from build123d import *

# Parameters (mm, degrees)
SKETCH1_W          = 110
SKETCH1_H          = 25
SKETCH2_W          = 16
SKETCH2_H          = 11.86901723
CUT_EXTRUDE1_DEPTH = 90
CHAMFER1_SIZE      = 2
FILLET1_R          = 3


with BuildPart() as part:
    # Sketch1 → Revolve1 (revolve)
    with BuildSketch(Plane.XY, mode=Mode.PRIVATE) as revolve1_sk:
        with Locations((0, 12.5)):
            Rectangle(SKETCH1_W, SKETCH1_H)
    revolve(revolve1_sk.sketch.rotate(Axis((-55, 0, 0), (1, 0, 0)), 90), axis=Axis((-55, 0, 0), (1, 0, 0)))

    # Sketch2 → Cut-Extrude1 (cut)
    with BuildSketch(Plane(origin=(55, 0, 0), x_dir=(0, 0, -1), z_dir=(1, 0, 0))):
        with Locations((0, 24.934508615)):
            Rectangle(SKETCH2_W, SKETCH2_H)
    extrude(amount=-CUT_EXTRUDE1_DEPTH, mode=Mode.SUBTRACT)

    # Chamfer1
    chamfer1_edges = [part.edges().sort_by_distance(p)[0] for p in [
        (55, -20.310096012, -14.577379737),
    ]]
    chamfer(chamfer1_edges, length=CHAMFER1_SIZE)

    # Fillet1
    fillet1_edges = [part.edges().sort_by_distance(p)[0] for p in [
        (-35, 19, 0),
    ]]
    fillet(fillet1_edges, radius=FILLET1_R)


solid = part.part
Build history of the part. All positions in model axes, mm. A direction names the side the tool comes from. Coordinates: 2 decimals unless noted, no trailing zeros. Write each loop counter-clockwise with the first axis right and the second up, starting at its lowest first coordinate (ties: lowest second). Pieces come first, ordered by that corner, then holes. Notation, with made-up numbers: (32, 0.25) -> (38, 0.25) arc R23 cw to (38, 8.25) -> close; hole circle Ø3 at (63, 13.5). An arc over 180 degrees is marked (long way). Use CSV: the item, a comma, the result in double quotes. Start each with the question number.
Q1. Cut at A-A, the plane z = 0. List the corners of the cut face in (x, y), then the cut area to 3 significant figures.
Q2. Cut at B-B, the plane x = 5. List the corners of the cut face in (y, z).
Q3. Pull direction Z, two halves, no side cores. Call faces 3 (the flat face through (11, 21, -8)), 4 (the conical face through (54.68, -23.3, 0.92)), 5 (the flat face through (55, -1, 0)), 6 (the flat face through (-35, 23, 0)): released by +Z, released by -Z, zero draft, split by the parting line, or undercut.
Q4. 3-axis set-ups, long thin cutter, end or side, ignore diameter. For faces 1 (the cylindrical face through (-0.244, -24.787, -3.255)), 2 (the flat face through (12, 19, 0)): which of +Z, -Z, +X, -X, +Y, -Y reach the whole face in a straight line?
Q5. Flat gauge pins, fed straight in: pin 1 Ø6 at (x, y) = (0.5, 13.5) entering from +Z; pin 2 Ø4 at (x, z) = (-20.5, 1) entering from +Y; pin 3 Ø2.5 at (x, y) = (31, 21) entering from -Z. Where does each tip first touch, or does it go through?
Q6. Drill centre lines: probe 1 along Z at (x, y) = (-1.5, 1); probe 2 along Y at (x, z) = (34, 20); probe 3 along Z at (x, y) = (-45, -5). Where is each one in solid material? Low to high.
Q7. Cut at C-C, the plane x = -37.5. List the corners of the cut face in (y, z), then the cut area to 3 significant figures.
Checked values:
1,outline,"(-55, -25) -> (53, -25) -> (55, -23) -> (55, 19) -> (-32, 19) arc R3 cw to (-35, 22) -> (-35, 25) -> (-55, 25) -> close"
1,area,"4,960 mm²"
2,outline,"(19, -8) -> (19, 8) -> (23.69, 8) arc R25 ccw (long way) to (23.69, -8) -> close"
3,face 3,"undercut"
3,face 4,"split by the parting line"
3,face 5,"zero draft"
3,face 6,"undercut"
4,face 1,"+X, -X"
4,face 2,"+X, +Y"
5,pin 1,"stops at z = 22.69"
5,pin 2,"stops at y = 19"
5,pin 3,"stops at z = -15.33"
6,probe 1,"z = -24.98 to 24.98"
6,probe 2,"y = -15 to 15"
6,probe 3,"z = -24.49 to 24.49"
7,outline,"circle Ø50 at (0, 0)"
7,area,"1,960 mm²"
